```python
from build123d import *

# Parameters (mm, degrees)
F0_W     = 77.51
F0_H     = 77.519
F0_R     = 2.55
F0_W_2   = 29.902
F0_H_2   = 29.9
F0_R_2   = 5
F1_DEPTH = 12
F2_DEPTH = 6
F3_R     = 5


with BuildPart() as f1:
    # F0 (on Top) → F1 (new body)
    with BuildSketch(Plane.XY):
        Rectangle(F0_W, F0_H)
        with Locations((-30, -29.9995)):
            Circle(F0_R, mode=Mode.SUBTRACT)
        with Locations((30, -29.9995)):
            Circle(F0_R, mode=Mode.SUBTRACT)
        with Locations((-30, 29.9995)):
            Circle(F0_R, mode=Mode.SUBTRACT)
        Rectangle(F0_W_2, F0_H_2, mode=Mode.SUBTRACT)
        with Locations((30, 29.9995)):
            Circle(F0_R, mode=Mode.SUBTRACT)
        Rectangle(F0_W_2, F0_H_2)
        Circle(F0_R_2, mode=Mode.SUBTRACT)
    extrude(amount=F1_DEPTH)

    # F0 (on Top) → F2 (cut)
    with BuildSketch(Plane.XY):
        Rectangle(F0_W_2, F0_H_2)
        Circle(F0_R_2, mode=Mode.SUBTRACT)
    extrude(amount=F2_DEPTH, mode=Mode.SUBTRACT)

    # F3
    f3_edges = [f1.edges().sort_by_distance(p)[0] for p in [
        (38.755, -38.7595, 6),
        (-38.755, -38.7595, 6),
        (38.755, 38.7595, 6),
        (-38.755, 38.7595, 6),
    ]]
    fillet(f3_edges, radius=F3_R)


solid = f1.part
```
Design review of the part built by this model. Coordinates are the model's own, in mm. A direction names the side the tool comes from. Give positions to 0.01 mm unless a question says otherwise; leave off trailing zeros. Loops run counter-clockwise (first coordinate to the right, second up) from the corner with the lowest first, then second, coordinate; pieces in that order, holes last. Notation, with made-up numbers: (60, 24) -> (76, 24) arc R13 cw to (76, 48) -> close; hole circle Ø3 at (22.25, 79.25). An arc over 180 degrees is marked (long way). One line per item, written item: value.
Q1. We need section A-A on x = 3. Give the boundary of the cut face in (y, z), and give its area (3 significant figures).
Numbers:
outline: (-38.76, 0) -> (-14.95, 0) -> (-14.95, 6) -> (-4, 6) -> (-4, 12) -> (-38.76, 12) -> close; (4, 6) -> (14.95, 6) -> (14.95, 0) -> (38.76, 0) -> (38.76, 12) -> (4, 12) -> close
area: 703 mm^2
Q2. We need section C-C on y = 0. Give the boundary of the cut face in (x, z) (3 decimals), and give its area (3 significant figures).
Numbers:
outline: (-38.755, 0) -> (-14.951, 0) -> (-14.951, 6) -> (-5, 6) -> (-5, 12) -> (-38.755, 12) -> close; (5, 6) -> (14.951, 6) -> (14.951, 0) -> (38.755, 0) -> (38.755, 12) -> (5, 12) -> close
area: 691 mm^2
Q3. For pin 1 Ø11.5 at (x, y) = (0, 0) entering from -Z, flat-tipped, find the tip position at first contact; note if it passes through.
Numbers:
pin 1: stops at z = 6
Q4. We need section D-D on z = 5. Give the number of separate pieces and of enclosed holes in the cut face, and give its area (3 significant figures).
Numbers:
separate pieces: 1
enclosed holes: 5
area: 5,010 mm^2
Q5. We need section B-B on x = -30. Give the boundary of the cut face in (y, z).
Numbers:
outline: (-38.76, 0) -> (-32.55, 0) -> (-32.55, 12) -> (-38.76, 12) -> close; (-27.45, 0) -> (27.45, 0) -> (27.45, 12) -> (-27.45, 12) -> close; (32.55, 0) -> (38.76, 0) -> (38.76, 12) -> (32.55, 12) -> close
Q6. For L1, parallel to Y at x = 30, z = 9; L2, parallel to X at y = -3.5, z = 0.5 (3 decimals); L3, parallel to Y at x = -1, z = 1.25, list the stretches that pass through material, from the lowest coordinate up.
Numbers:
L1: y = -38.76 to -32.55, -27.45 to 27.45, 32.55 to 38.76
L2: x = -38.755 to -14.951, 14.951 to 38.755
L3: y = -38.76 to -14.95, 14.95 to 38.76
Q7. Machinability: for faces 1 (the flat face through (14.951, 0, 3)), 2 (the cylindrical face through (37.251, 37.334, 6.084)), which of the approach directions +Z, -Z, +X, -X, +Y, -Y give a long, thin tool a straight path to every point of the face, cutting with its end or side? Answer none if there is none.
Numbers:
face 1: -Z
face 2: +Z, -Z, +X, +Y
